Source: CAD feature listing. Evaluate the final solid. Frame: model axes, mm. Face numbers are marked on the shaded views. A direction names the side the tool comes from. Give positions to 0.01 mm unless a question says otherwise; leave off trailing zeros. Order: outer loops, then holes, each group sorted by start corner. A loop starts at its lowest first (then second) coordinate and runs counter-clockwise, first axis right, second up. Notation, with made-up numbers: M -4,80 L 40,80 A3 ccw 40,85 Z; hole C 57.5,79.5 d9. An arc over 180 degrees is marked long. Answer in a Markdown table with one row per item. Add a question column.
(1) Set-up query: the marked faces 1, 2 and 3. Return all of +Z, -Z, +X, -X, +Y, -Y with unobstructed straight access to the full face (end or side cutting, diameter ignored); none if empty.
(2) Material intervals for line 1 along Y through (x, z) = (6, -0.5); line 2 along X through (y, z) = (-1.25, 0); line 3 along Y through (x, z) = (-6.5, 0.5), sorted ascending.
(3) Mould query, pull axis X, two halves, no side actions, for the marked faces 4, 5, 6 and 7. Classes: pulls with the +X half, pulls with the -X half, needs draft (parallel to the pull), parting line crosses it, or undercut.
(4) Section query D-D, the plane z = -2. Return loops of the section in (x, y), plus the area to 3 significant figures.
(5) Section query B-B, the plane z = 0. Return loops of the section in (x, y).
(6) Section query A-A, the plane y = 2.75. Return loops of the section in (x, z) (1 decimal).
(7) Pin query (flat end, axial travel): P1, Ø4, axis at x = 3.5, z = -2, coming from the -Y side; P2, Ø5, axis at x = -1.5, z = -2, coming from the +Y side. Return the tip coordinate at first contact, or that it passes through.
(8) Section query C-C, the plane x = -9.5. Return loops of the section in (y, z), plus the area to 3 significant figures.
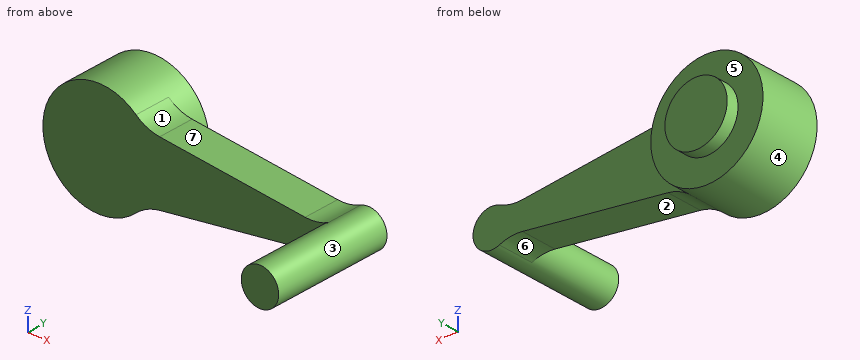
from build123d import *

# Parameters (mm, degrees)
SKETCH1_R                = 4.5
BOSS_EXTRUDE1_DEPTH      = 5
SKETCH1_3_R              = 1.5
BOSS_EXTRUDE2_DEPTH      = 3
BOSS_EXTRUDE2_DEPTH_BACK = 7
BOSS_EXTRUDE3_DEPTH      = 3
SKETCH3_R                = 2.5
BOSS_EXTRUDE4_DEPTH      = 1


with BuildPart() as part:
    # Sketch1 → Boss-Extrude1 (new body)
    with BuildSketch(Plane(origin=(0, 0, 0), x_dir=(1, 0, 0), z_dir=(0, 1, 0))):
        with Locations((-9.5, 0)):
            Circle(SKETCH1_R)
    extrude(amount=BOSS_EXTRUDE1_DEPTH)



with BuildPart() as body_2:
    # Sketch1_3 → Boss-Extrude2 (new body, two sides)
    with BuildSketch(Plane(origin=(0, 0, 0), x_dir=(1, 0, 0), z_dir=(0, 1, 0))) as boss_extrude2_sk:
        with Locations((9.5, 0)):
            Circle(SKETCH1_3_R)
    extrude(amount=BOSS_EXTRUDE2_DEPTH)
    extrude(boss_extrude2_sk.sketch, amount=-BOSS_EXTRUDE2_DEPTH_BACK)


with BuildPart() as part_1:
    add(part.part)

    add(body_2.part)  # Boss-Extrude3 merges body 2
    # Sketch2 → Boss-Extrude3 (add)
    with BuildSketch(Plane(origin=(0, 0, 0), x_dir=(1, 0, 0), z_dir=(0, 1, 0))):
        with BuildLine():
            Line((-4.63504008, 2.526088469), (7.037637478, 1.092863881))
            ThreePointArc((7.037637478, 1.092863881), (7.982322779, 1.105340991), (8.889254054, 1.370032623))
            ThreePointArc((8.889254054, 1.370032623), (8, 0), (8.889254054, -1.370032623))
            ThreePointArc((8.889254054, -1.370032623), (7.982322779, -1.105340991), (7.037637478, -1.092863881))
            Line((7.037637478, -1.092863881), (-4.63504008, -2.526088469))
            ThreePointArc((-4.63504008, -2.526088469), (-5.643496055, -2.807700077), (-6.523529775, -3.375))
            ThreePointArc((-6.523529775, -3.375), (-5, 0), (-6.523529775, 3.375))
            ThreePointArc((-6.523529775, 3.375), (-5.643496055, 2.807700077), (-4.63504008, 2.526088469))
        make_face()
    extrude(amount=BOSS_EXTRUDE3_DEPTH)

    # Sketch3 → Boss-Extrude4 (add)
    with BuildSketch(Plane(origin=(0, 5, 0), x_dir=(1, 0, 0), z_dir=(0, 1, 0))):
        with Locations((-9.5, 0)):
            Circle(SKETCH3_R)
    extrude(amount=BOSS_EXTRUDE4_DEPTH)


solid = part_1.part
Values follow:
| question | item | result |
|---|---|---|
| 1 | face 1 | +Z, +X, +Y, -Y |
| 1 | face 2 | -Z, +Y, -Y |
| 1 | face 3 | -Y |
| 2 | line 1 | y = 0 to 3 |
| 2 | line 2 | x = 8 to 11 |
| 2 | line 3 | y = 0 to 5 |
| 3 | face 4 | parting line crosses it |
| 3 | face 5 | needs draft |
| 3 | face 6 | undercut |
| 3 | face 7 | undercut |
| 4 | outline | M -13.53,0 L -0.35,0 L -0.35,3 L -5.47,3 L -5.47,5 L -8,5 L -8,6 L -11,6 L -11,5 L -13.53,5 Z |
| 4 | area | 58.7 mm² |
| 5 | outline | M -14,0 L 8,0 L 8,-7 L 11,-7 L 11,3 L -5,3 L -5,5 L -7,5 L -7,6 L -12,6 L -12,5 L -14,5 Z |
| 6 | outline | M -6.5,-3.4 A3.5 cw -4.6,-2.5 L 7,-1.1 A3.5 cw 8.9,-1.4 A1.5 ccw long 8.9,1.4 A3.5 cw 7,1.1 L -4.6,2.5 A3.5 cw -6.5,3.4 A4.5 ccw long Z |
| 7 | P1 | stops at y = 0 |
| 7 | P2 | stops at y = 3 |
| 8 | outline | M 0,-4.5 L 5,-4.5 L 5,-2.5 L 6,-2.5 L 6,2.5 L 5,2.5 L 5,4.5 L 0,4.5 Z |
| 8 | area | 50.0 mm² |
